Input: part model. Units: mm. Frame: model coordinates. Round coordinates to 2 decimals unless told otherwise and drop trailing zeros. Loops run counter-clockwise (first coordinate to the right, second up) from the corner with the lowest first, then second, coordinate; pieces in that order, holes last. Notation, with made-up numbers: M 9,-10 L 65,-10 A19 cw 65,15 Z; hole C -13.5,-3.75 d4. An arc over 180 degrees is marked long. Return JSON: item names as keys, results as strings. Group by question number.
1) Material intervals for line 1 (X direction, y = 9, z = 1.8); line 2 (X direction, y = 26, z = -0.25); line 3 (Y direction, x = 17, z = 0.3), sorted ascending. Write a range as from..to.
2) Section B-B (x = 25). Output: boundary loops of the cut face in (y, z), plus the area to 3 significant figures.
3) Section A-A (y = 16). Output: boundary loops of the cut face in (x, z).
4) Section C-C (z = 1.6). Output: boundary loops of the cut face in (x, y), plus the area to 3 significant figures.
5) Contact query for flat-ended pins moving along their axis: P1, Ø4, axis at x = 40.65, y = -35.05, coming from the -Z side; P2, Ø1.5, axis at y = -9.5, z = 1.5, coming from the -X side; P3, Ø1.1, axis at x = -17, z = -0.5, coming from the -Y side. Output: stop coordinate, or through.
Autodesk Inventor part; units mm, degrees
ref_plane "YZ Plane" through (0, 0, 0) normal (1, 0, 0) x (0, 1, 0)
ref_plane "XZ Plane" through (0, 0, 0) normal (0, 1, 0) x (-1, 0, 0)
ref_plane "XY Plane" through (0, 0, 0) normal (0, 0, 1) x (1, 0, 0)
sketch "Skizze1" plane through (0, 0, 0) normal (0, 0, 1) x (1, 0, 0)
  line L0 (-41, 29.8031) -> (-41, -33.4)
  arc A0 (-36.9771, 35.8002) -> (-42.1832, 31.6287) centre (-40.6517, 35.0517) ccw
  arc A1 (-41, 29.8031) -> (-42.1832, 31.6287) centre (-43, 29.8031) ccw
  line L1 (-23, 35.4) -> (-36.4872, 35.4)
  arc A2 (-36.9771, 35.8002) -> (-36.4872, 35.4) centre (-36.4872, 35.9) ccw
  line L2 (39, 35.4) -> (-8, 35.4)
  line L3 (41, -29.8031) -> (41, 33.4)
  arc A3 (41, 33.4) -> (39, 35.4) centre (39, 33.4) ccw
  circle A4 centre (-40.6517, 35.0517) radius 1.25
  circle A5 centre (40.6517, -35.0517) radius 1.25
  arc A6 (36.9771, -35.8002) -> (42.1832, -31.6287) centre (40.6517, -35.0517) ccw
  arc A7 (41, -29.8031) -> (42.1832, -31.6287) centre (43, -29.8031) ccw
  arc A8 (36.9771, -35.8002) -> (36.4872, -35.4) centre (36.4872, -35.9) ccw
  line L4 (35, -35.4) -> (36.4872, -35.4)
  arc A9 (-41, -33.4) -> (-39, -35.4) centre (-39, -33.4) ccw
  line L5 (-39, -35.4) -> (-35, -35.4)
  line L6 (-35, -35.4) -> (35, -35.4)
  line L7 (-23, 35.4) -> (-8, 35.4)
  circle A10 centre (40.6517, -35.0517) radius 1.7
  circle A11 centre (-40.6517, 35.0517) radius 1.7
  point P0 (0, 0)
  point P1 (-36.651, 36.3964)
  dimension "d6" = 3.4
extrude "Extrusion1" add sketch "Skizze1" along normal blind 3 contours A1 A0 A2 L1 L7 L2 A3 L3 A7 A6 A8 L4 L6 L5 A9 L0
ref_plane "Arbeitsebene1" through (0, 0, 0) normal (0, 0, -1) x (-1, 0, 0)
sketch "Skizze2" plane through (0, 0, 0) normal (0, 0, -1) x (-1, 0, 0)
  line L0 (-38, 32.1) -> (-38, -32.1)
  line L1 (33, -32.4) -> (-33, -32.4)
  line L2 (-37.7, -32.4) -> (-33, -32.4)
  arc A0 (-38, -32.1) -> (-37.7, -32.4) centre (-37.7, -32.1) ccw
  line L3 (-33, 32.4) -> (33, 32.4)
  line L4 (-33, 32.4) -> (-37.7, 32.4)
  arc A1 (-37.7, 32.4) -> (-38, 32.1) centre (-37.7, 32.1) ccw
  line L5 (38, -32.1) -> (38, 32.1)
  line L6 (33, -32.4) -> (37.7, -32.4)
  arc A2 (37.7, -32.4) -> (38, -32.1) centre (37.7, -32.1) ccw
  line L7 (37.7, 32.4) -> (33, 32.4)
  arc A3 (38, 32.1) -> (37.7, 32.4) centre (37.7, 32.1) ccw
  line L8 (-32.5, -32.2) -> (32.5, -32.2)
  line L9 (32.5, -32.2) -> (35.8, -32.2)
  line L10 (37.8, -30.2) -> (37.8, 31.2)
  line L11 (36.8, 32.2) -> (32.5, 32.2)
  line L12 (32.5, 32.2) -> (-32.5, 32.2)
  line L13 (-32.5, 32.2) -> (-36.8, 32.2)
  line L14 (-37.8, 31.2) -> (-37.8, -31.2)
  line L15 (-36.8, -32.2) -> (-32.5, -32.2)
  arc A4 (35.8, -32.2) -> (37.8, -30.2) centre (35.8, -30.2) ccw
  arc A5 (37.8, 31.2) -> (36.8, 32.2) centre (36.8, 31.2) ccw
  arc A6 (-36.8, 32.2) -> (-37.8, 31.2) centre (-36.8, 31.2) ccw
  arc A7 (-37.8, -31.2) -> (-36.8, -32.2) centre (-36.8, -31.2) ccw
  point P0 (37.8, -32.2)
  point P1 (37.8, 32.2)
  point P2 (-37.8, 32.2)
  point P3 (-37.8, -32.2)
  dimension "d7" = 0.2
  dimension "d8" = 2
  dimension "d9" = 1
extrude "Extrusion2" add sketch "Skizze2" along normal blind 1 contours L15 A7 L14 A6 L13 L12 L11 A5 L10 A4 L9 L8
properties part number "deckel"
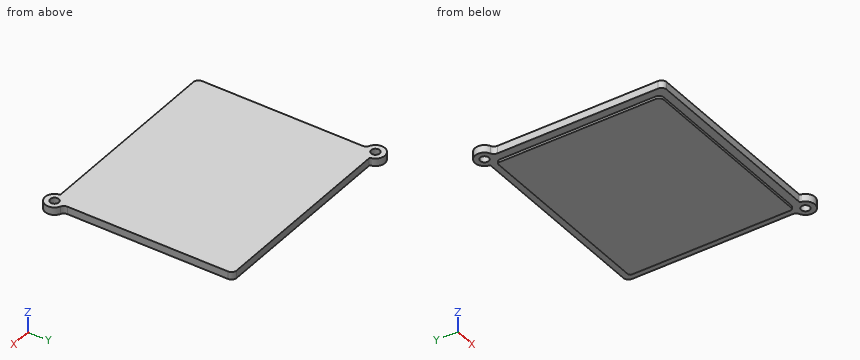
Returned:
{
 "1": {"line 1": "x = -41..41", "line 2": "x = -37.8..37.8", "line 3": "y = -35.4..35.4"},
 "2": {"outline": "M -35.4,0 L -32.2,0 L -32.2,-1 L 32.2,-1 L 32.2,0 L 35.4,0 L 35.4,3 L -35.4,3 Z", "area": "277 mm^2"},
 "3": {"outline": "M -41,0 L -37.8,0 L -37.8,-1 L 37.8,-1 L 37.8,0 L 41,0 L 41,3 L -41,3 Z"},
 "4": {"outline": "M -42.18,31.63 A2 cw -41,29.8 L -41,-33.4 A2 ccw -39,-35.4 L 36.49,-35.4 A0.5 cw 36.98,-35.8 A3.75 ccw long 42.18,-31.63 A2 cw 41,-29.8 L 41,33.4 A2 ccw 39,35.4 L -36.49,35.4 A0.5 cw -36.98,35.8 A3.75 ccw long Z; hole C -40.65,35.05 d3.4; hole C 40.65,-35.05 d3.4", "area": "5,850 mm^2"},
 "5": {"P1": "stops at z = 0", "P2": "stops at x = -41", "P3": "stops at y = -35.4"}
}
